Could you check a few things on this model? Use its own coordinates, in mm. A direction names the side the tool comes from. Give positions to 0.01 mm unless a question says otherwise; leave off trailing zeros. Write each loop counter-clockwise with the first axis right and the second up, starting at its lowest first coordinate (ties: lowest second). Pieces come first, ordered by that corner, then holes. Notation, with made-up numbers: M 88,85.25 L 100,85.25 A21 ccw 100,124.25 Z; hole C 26.5,-20 d9. An arc over 180 degrees is marked long. Answer as a JSON object with one key per item and string values. Group by question number.
Autodesk Inventor part; units mm, degrees
ref_plane "YZ Plane" through (0, 0, 0) normal (1, 0, 0) x (0, 1, 0)
ref_plane "XZ Plane" through (0, 0, 0) normal (0, 1, 0) x (-1, 0, 0)
ref_plane "XY Plane" through (0, 0, 0) normal (0, 0, 1) x (1, 0, 0)
sketch "Sketch1" plane through (0, 0, 0) normal (0, 0, 1) x (1, 0, 0)
  line L0 (0, 0) -> (41.5, 0)
  line L1 (41.5, 0) -> (41.5, -73)
  line L2 (41.5, -73) -> (0, -73)
  line L3 (0, -73) -> (0, 0)
  line L4 (0, -73) -> (3.11, -73)
  line L5 (0, -73) -> (3.11, -73) construction
  line L6 (3.11, -73) -> (3.11, -69.85)
  line L7 (3.11, -73) -> (6.26, -73) construction
  line L8 (3.11, -69.85) -> (14.54, -69.85)
  line L9 (14.54, -69.85) -> (19.65, -69.85)
  line L10 (19.65, -69.85) -> (31.08, -69.85)
  circle A0 centre (3.11, -69.85) radius 1.6
  circle A1 centre (14.54, -69.85) radius 1.6
  circle A2 centre (19.65, -69.85) radius 1.6
  circle A3 centre (31.08, -69.85) radius 1.6
  line L11 (3.11, -69.85) -> (3.11, -55.42)
  line L12 (3.11, -69.85) -> (17.54, -69.85) construction
  line L13 (0, -73) -> (4.33, -73)
  line L14 (0, -73) -> (4.33, -73) construction
  line L15 (4.33, -73) -> (4.33, -53.49)
  line L16 (3.11, -55.42) -> (6.6479, -55.42)
  circle A4 centre (4.33, -55.42) radius 1.651
  line L17 (4.33, -55.42) -> (4.33, -37.69)
  line L18 (4.33, -55.42) -> (22.06, -55.42) construction
  line L19 (4.33, -55.42) -> (29.68, -55.42)
  line L20 (4.33, -55.42) -> (29.68, -55.42) construction
  circle A5 centre (4.33, -37.69) radius 1.651
  circle A6 centre (29.68, -55.42) radius 1.651
  line L21 (4.33, -37.69) -> (39.0376, -37.69)
  line L22 (29.68, -55.42) -> (29.68, -25.3245)
  circle A7 centre (29.68, -37.69) radius 1.651
  line L23 (4.33, -37.69) -> (4.33, -30.44)
  line L24 (4.33, -37.69) -> (11.58, -37.69) construction
  line L25 (4.33, -30.44) -> (4.33, -12.71)
  line L26 (4.33, -30.44) -> (29.68, -30.44)
  line L27 (4.33, -30.44) -> (29.68, -30.44) construction
  line L28 (4.33, -12.71) -> (29.68, -12.71)
  circle A8 centre (29.48, -12.71) radius 1.651
  circle A9 centre (4.33, -12.71) radius 1.651
  circle A10 centre (4.33, -30.44) radius 1.651
  circle A11 centre (29.68, -30.44) radius 1.651
  dimension "d0" = 41.5
  dimension "d1" = 73
  dimension "d2" = 3.11
  dimension "d3" = 0
  dimension "d4" = 3.15
  dimension "d5" = 90
  dimension "d6" = 11.43
  dimension "d7" = 90
  dimension "d9" = 5.11
  dimension "d10" = 11.43
  dimension "d11" = 180
  dimension "d12" = 3.2
  dimension "d13" = 3.2
  dimension "d14" = 3.2
  dimension "d15" = 3.2
  dimension "d18" = 14.43
  dimension "d19" = 90
  dimension "d20" = 4.33
  dimension "d21" = 0
  dimension "d22" = 3.302
  dimension "d23" = 17.73
  dimension "d24" = 90
  dimension "d25" = 25.35
  dimension "d26" = 0
  dimension "d27" = 3.302
  dimension "d28" = 3.302
  dimension "d29" = 3.302
  dimension "d30" = 7.25
  dimension "d31" = 90
  dimension "d32" = 17.73
  dimension "d33" = 180
  dimension "d34" = 25.35
  dimension "d35" = 0
  dimension "d36" = 25.35
  dimension "d37" = 3.302
  dimension "d38" = 3.302
  dimension "d39" = 3.302
  dimension "d40" = 3.302
extrude "Extrusion2" add sketch "Sketch1" along normal blind 2 contours L0 L1 L2 L15 A0 A4 L16 L19 A6 L22 A7 A11 L26 A10 L23 A5 L17 L11 L6 L3 | L6 A0 L15 L2 | L11 A4 L15 A0 | L15 L17 A5 L21 A7 L22 A6 L19 L16 A4 | L23 A10 L26 A11 L22 A7 L21 A5
sketch "Sketch3" plane through (0, 0, 2) normal (0, 0, 1) x (1, 0, 0)
  circle A0 centre (4.33, -55.42) radius 1.651
  circle A1 centre (4.33, -55.42) radius 3.5
  circle A2 centre (29.68, -55.42) radius 1.651
  circle A3 centre (29.68, -55.42) radius 3.5
  circle A4 centre (4.33, -12.71) radius 1.651
  circle A5 centre (4.33, -12.71) radius 3.5
  circle A6 centre (29.48, -12.71) radius 1.651
  circle A7 centre (29.48, -12.71) radius 3.5
  point P0 (0, 0)
  dimension "d46" = 7
  dimension "d47" = 7
  dimension "d48" = 7
  dimension "d49" = 7
extrude "Extrusion4" add sketch "Sketch3" along normal blind 10
sketch "Sketch8" plane through (0, 0, 0) normal (0, 0, -1) x (-1, 0, 0)
  circle A0 centre (-4.33, -12.71) radius 1.651
  circle A1 centre (-4.33, -12.71) radius 12.71
  line L0 (-41.5, 0) -> (0, 0)
  line L1 (8.38, -12.71) -> (8.38, -69.4926)
  circle A2 centre (-4.33, -55.42) radius 1.651
  circle A3 centre (-4.33, -55.42) radius 12.71
  circle A4 centre (-4.33, -55.42) radius 4.33
  circle A5 centre (-4.33, -12.71) radius 4.33
  line L2 (0, -55.42) -> (0, -59.75)
  line L3 (0, -59.75) -> (-4.33, -59.75)
  line L4 (0, 0) -> (0, -73)
  line L5 (0, -12.71) -> (0, -8.38)
  line L6 (0, -8.38) -> (-4.33, -8.38)
  line L7 (0, -8.38) -> (-8.66, -8.38)
  line L8 (-8.66, -8.38) -> (-8.66, -59.75)
  line L9 (-8.66, -59.75) -> (0, -59.75)
  line L10 (0, -59.75) -> (0, -8.38)
  circle A6 centre (-4.33, -12.71) radius 1.651
  circle A7 centre (-4.33, -55.42) radius 1.651
extrude "Extrusion5" add sketch "Sketch8" along normal blind 10 contours L4 A3 L8 A1 | A1 L8 A5 L4 | L4 A5 L6 | A5 | L4 A4 L8 A3 | A5 L8 L7 | L2 L3 A4 | A4 | A4 L9 L8
sketch "Sketch9" plane through (8.66, -59.75, 0) normal (1, 0, 0) x (0, 0, -1)
  line L0 (10, 0) -> (10, 51.37)
  line L1 (10, 25.685) -> (0, 25.685)
  line L2 (0, 25.685) -> (0, 35.685)
  line L3 (0, 35.685) -> (10, 35.685)
  line L4 (10, 35.685) -> (10, 25.685)
  line L5 (10, 25.685) -> (0, 25.685)
  line L6 (0, 25.685) -> (0, 15.685)
  line L7 (0, 15.685) -> (10, 15.685)
  line L8 (10, 15.685) -> (10, 25.685)
  line L9 (10, 25.685) -> (0, 35.685)
  line L10 (10, 25.685) -> (0, 15.685)
  line L11 (0, 51.37) -> (10, 51.37)
  line L12 (10, 51.37) -> (0, 51.37)
  line L13 (0, 51.37) -> (0, 41.37)
  line L14 (0, 41.37) -> (10, 41.37)
  line L15 (10, 41.37) -> (10, 51.37)
  line L16 (10, 0) -> (0, 0)
  line L17 (0, 0) -> (0, 10)
  line L18 (0, 10) -> (10, 10)
  line L19 (10, 10) -> (10, 0)
  line L20 (10, 41.37) -> (0, 41.37)
  line L21 (0, 41.37) -> (0, 10)
  line L22 (0, 10) -> (10, 10)
  line L23 (10, 10) -> (10, 41.37)
  point P0 (0, 59.75)
  dimension "d55" = 10
  dimension "d56" = 10
  dimension "d57" = 10
  dimension "d58" = 10
  dimension "d59" = 10
  dimension "d60" = 10
  dimension "d61" = 10
  dimension "d62" = 10
extrude "Extrusion6" cut sketch "Sketch9" against normal blind 5 contours L18 L21 L7 L0 | L7 L10 L0 | L9 L3 L0 | L10 L6 L1 | L1 L2 L9 | L3 L21 L14 L0
sketch "Sketch11" plane through (3.66, -59.75, 0) normal (1, 0, 0) x (0, 0, -1)
  line L0 (10, 51.37) -> (10, 41.37)
  line L1 (10, 41.37) -> (0, 41.37)
  line L2 (0, 41.37) -> (0, 31.37)
  line L3 (0, 31.37) -> (10, 31.37)
  line L4 (10, 31.37) -> (10, 41.37)
  line L5 (10, 41.37) -> (10, 10)
  line L6 (10, 25.685) -> (0, 25.685)
  line L7 (0, 25.685) -> (0, 35.685)
  line L8 (0, 35.685) -> (10, 35.685)
  line L9 (10, 35.685) -> (10, 25.685)
  line L10 (10, 25.685) -> (0, 25.685)
  line L11 (0, 25.685) -> (0, 35.685)
  line L12 (0, 35.685) -> (10, 35.685)
  line L13 (10, 35.685) -> (10, 25.685)
  line L14 (10, 25.685) -> (0, 25.685)
  line L15 (0, 25.685) -> (0, 15.685)
  line L16 (0, 15.685) -> (10, 15.685)
  line L17 (10, 15.685) -> (10, 25.685)
  line L18 (10, 25.685) -> (0, 35.685)
  line L19 (10, 25.685) -> (0, 15.685)
  circle A0 centre (5, 30.685) radius 1.651
  circle A1 centre (5, 20.685) radius 1.651
  point P0 (0, 59.75)
  dimension "d65" = 10
  dimension "d66" = 10
  dimension "d67" = 10
  dimension "d68" = 10
  dimension "d69" = 10
  dimension "d70" = 10
  dimension "d71" = 10
  dimension "d72" = 10
  dimension "d73" = 3.302
  dimension "d74" = 3.302
extrude "Extrusion7" cut sketch "Sketch11" against normal blind 5 contours A0 L3 L18 | L18 L3 A0 | A0 L18 L3 | L3 L18 A0 | A1 L19 | L19 A1
sketch "Sketch12" plane through (0, 0, 0) normal (0, 0, -1) x (-1, 0, 0)
  line L0 (-41.5, -73) -> (-41.5, 0)
  line L1 (-41.5, -73) -> (0, -73)
  line L2 (0, -73) -> (0, 0)
  line L3 (0, 0) -> (-41.5, 0)
  line L4 (-41.5, 0) -> (-41.5, -73)
extrude "Extrusion8" cut sketch "Sketch12" against normal blind 30
sketch "Sketch14" plane through (3.66, -59.75, 0) normal (1, 0, 0) x (0, 0, -1)
  point P0 (0, 59.75)
sketch "Sketch15" plane through (0, 0, -10) normal (0, 0, -1) x (-1, 0, 0)
  circle A0 centre (-4.33, -55.42) radius 1.651
  circle A1 centre (-4.33, -55.42) radius 1.651
  circle A2 centre (-4.33, -12.71) radius 1.651
  circle A3 centre (-4.33, -12.71) radius 1.651
  circle A4 centre (-4.33, -12.71) radius 3
  circle A5 centre (-4.33, -55.42) radius 3
  line L0 (-7.33, -55.42) -> (-5.83, -52.8219)
  line L1 (-5.83, -52.8219) -> (-2.83, -52.8219)
  line L2 (-2.83, -52.8219) -> (-1.33, -55.42)
  line L3 (-1.33, -55.42) -> (-2.83, -58.0181)
  line L4 (-2.83, -58.0181) -> (-5.83, -58.0181)
  line L5 (-5.83, -58.0181) -> (-7.33, -55.42)
  line L6 (-7.33, -12.71) -> (-5.83, -10.1119)
  line L7 (-5.83, -10.1119) -> (-2.83, -10.1119)
  line L8 (-2.83, -10.1119) -> (-1.33, -12.71)
  line L9 (-1.33, -12.71) -> (-2.83, -15.3081)
  line L10 (-2.83, -15.3081) -> (-5.83, -15.3081)
  line L11 (-5.83, -15.3081) -> (-7.33, -12.71)
  point P0 (0, 0)
  dimension "d79" = 6
  dimension "d80" = 6
extrude "Extrusion9" cut sketch "Sketch15" against normal blind 2 contours L9 L10 L11 L6 L7 L8 | L3 L4 L5 L0 L1 L2
sketch "Sketch16" plane through (3.66, -59.75, 0) normal (1, 0, 0) x (0, 0, -1)
  circle A0 centre (5, 20.685) radius 1.651
  circle A1 centre (5, 20.685) radius 3
  circle A2 centre (5, 30.685) radius 1.651
  circle A3 centre (5, 30.685) radius 3
  line L0 (5, 17.685) -> (2.4019, 19.185)
  line L1 (2.4019, 19.185) -> (2.4019, 22.185)
  line L2 (2.4019, 22.185) -> (5, 23.685)
  line L3 (5, 23.685) -> (7.5981, 22.185)
  line L4 (7.5981, 22.185) -> (7.5981, 19.185)
  line L5 (7.5981, 19.185) -> (5, 17.685)
  line L6 (5, 27.685) -> (2.4019, 29.185)
  line L7 (2.4019, 29.185) -> (2.4019, 32.185)
  line L8 (2.4019, 32.185) -> (5, 33.685)
  line L9 (5, 33.685) -> (7.5981, 32.185)
  line L10 (7.5981, 32.185) -> (7.5981, 29.185)
  line L11 (7.5981, 29.185) -> (5, 27.685)
  point P0 (0, 59.75)
  dimension "d83" = 6
  dimension "d84" = 6
extrude "Extrusion10" cut sketch "Sketch16" against normal blind 2 contours L4 L5 L0 L1 L2 L3 | L10 L11 L6 L7 L8 L9
properties part number "mountBrace"
1) If we section it at A-A, the plane x = 4.33: List the corners of the cut face in (y, z) for me, plus the area to 3 significant figures.
2) If we section it at C-C, the plane y = -11.5: List the corners of the cut face in (x, z) for me, plus the area to 3 significant figures.
3) If we section it at B-B, the plane z = -4: List the corners of the cut face in (x, y) for me, plus the area to 3 significant figures.
4) For faces 4 (the flat face through (2.674, -31.304, -6.317)), 5 (the flat face through (2.07, -56.7, -9.01)), 6 (the cylindrical face through (4.545, -14.347, -3.944)), 7 (the cylindrical face through (0.842, -40.677, -4.642)), 8 (the flat face through (6, -49.75, -5)), which set-ups out of +Z, -Z, +X, -X, +Y, -Y let a thin tool reach every point of the face, with its end or its side?
5) We'd pull the mould along Y, two halves only. Please class faces 1 (the flat face through (4, -8.38, -5)), 2 (the flat face through (3, -14, -8)), 3 (the flat face through (8.66, -55, -5)): released by +Y, released by -Y, zero draft, split by the parting line, or undercut.
6) If we section it at D-D, the plane y = -22.5: List the corners of the cut face in (x, z) for me, plus the area to 3 significant figures.
7) I'm going to push flat-ended pins straight in: pin 1 (1 mm diameter, centred on y = -34, z = -6.5, fed in from +X); pin 2 (4.5 mm diameter, centred on x = 4.33, y = -12.71, fed in from -Z). Where does each tip first touch, or does it pass through?
8) Please list where these lines run through material, in increasing order: line 1 along Y through (x, z) = (4.33, -3.75); line 2 along Y through (x, z) = (0.65, -5); line 3 along Y through (x, z) = (6, -9). Write a range as from..to.
Taken from the geometry:
{
 "1": {"outline": "M -59.75,-10 L -58.02,-10 L -58.02,-8 L -57.07,-8 L -57.07,0 L -59.75,0 Z; M -53.77,-8 L -52.82,-8 L -52.82,-10 L -49.75,-10 L -49.75,0 L -53.77,0 Z; M -18.38,-10 L -15.31,-10 L -15.31,-8 L -14.36,-8 L -14.36,0 L -18.38,0 Z; M -11.06,-8 L -10.11,-8 L -10.11,-10 L -8.38,-10 L -8.38,0 L -11.06,0 Z", "area": "126 mm²"},
 "2": {"outline": "M 0,-10 L 2.03,-10 L 2.03,-8 L 3.21,-8 L 3.21,0 L 0,0 Z; M 5.45,-8 L 6.63,-8 L 6.63,-10 L 8.66,-10 L 8.66,0 L 5.45,0 Z", "area": "59.4 mm²"},
 "3": {"outline": "M 0,-59.75 L 8.66,-59.75 L 8.66,-49.75 L 3.66,-49.75 L 3.66,-41.49 L 1.66,-41.49 L 1.66,-40.38 L 0,-40.38 Z; M 0,-37.75 L 1.66,-37.75 L 1.66,-36.64 L 3.66,-36.64 L 3.66,-31.49 L 1.66,-31.49 L 1.66,-30.38 L 0,-30.38 Z; M 0,-27.75 L 1.66,-27.75 L 1.66,-26.64 L 3.66,-26.64 L 3.66,-18.38 L 8.66,-18.38 L 8.66,-8.38 L 0,-8.38 Z; hole C 4.33,-55.42 d3.3; hole C 4.33,-12.71 d3.3", "area": "243 mm²"},
 "4": {"face 4": "+X", "face 5": "-Z", "face 6": "+Z, -Z", "face 7": "+X, -X", "face 8": "+Z, -Z, +X"},
 "5": {"face 1": "released by +Y", "face 2": "undercut", "face 3": "zero draft"},
 "6": {"outline": "M 0,-10 L 3.66,-10 L 3.66,0 L 0,0 Z", "area": "36.6 mm²"},
 "7": {"pin 1": "x = 3.66", "pin 2": "z = -8"},
 "8": {"line 1": "-59.75..-57.07, -53.77..-49.75, -18.38..-14.36, -11.06..-8.38", "line 2": "-59.75..-40.72, -37.41..-30.72, -27.41..-8.38", "line 3": "-59.75..-57.72, -53.12..-49.75, -18.38..-15.01, -10.41..-8.38"}
}
